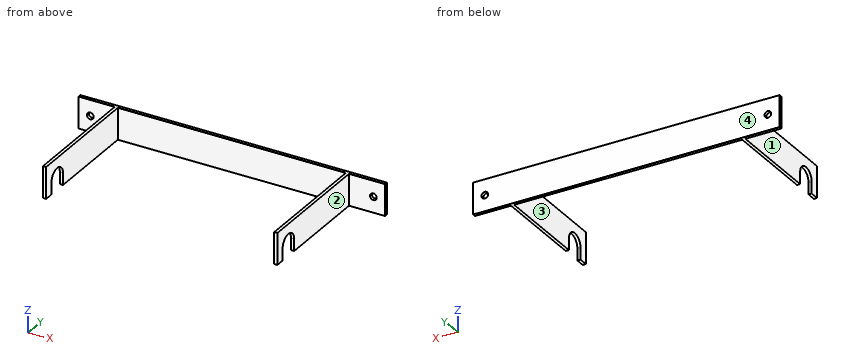
```python
from build123d import *

# Parameters (mm, degrees)
F0_W     = 390
F0_H     = 40
F0_R     = 4.25
F1_DEPTH = 4
F2_W     = 4
F2_H     = 40
F3_DEPTH = 155
F5_DEPTH = 298


with BuildPart() as f1:
    # F0 (on Front) → F1 (new body)
    with BuildSketch(Plane.XZ):
        with Locations((195, 20)):
            Rectangle(F0_W, F0_H)
        with Locations((15, 20)):
            Circle(F0_R, mode=Mode.SUBTRACT)
        with Locations((375, 20)):
            Circle(F0_R, mode=Mode.SUBTRACT)
    extrude(amount=F1_DEPTH)

    # F2 (on face) → F3 (join)
    with BuildSketch(Plane.XZ.offset(4)):
        with Locations((48, 20)):
            Rectangle(F2_W, F2_H)
        with Locations((342, 20)):
            Rectangle(F2_W, F2_H)
    extrude(amount=F3_DEPTH)

    # F4 (on face) → F5 (cut, through all)
    with BuildSketch(Plane.YZ.offset(344)):
        with BuildLine():
            Line((-122.5, 0), (-122.5, 15))
            ThreePointArc((-122.5, 15), (-135, 27.5), (-147.5, 15))
            Line((-147.5, 15), (-147.5, 0))
            Line((-147.5, 0), (-122.5, 0))
        make_face()
    extrude(amount=-F5_DEPTH, mode=Mode.SUBTRACT)


solid = f1.part
```
Part model, mm, in its own coordinate system. Face numbers are marked on the shaded views. A direction names the side the tool comes from. Round coordinates to 2 decimals unless told otherwise and drop trailing zeros. Order: outer loops, then holes, each group sorted by start corner. A loop starts at its lowest first (then second) coordinate and runs counter-clockwise, first axis right, second up. Notation, with made-up numbers: M 35,40.25 L 52,40.25 A28 ccw 52,59.25 Z; hole C 34,41.5 d10. An arc over 180 degrees is marked long. Answer in a Markdown table with one row per item. Add a question column.
Q1. Cut at D-D on z = 32. Give the cut face in (x, y), and give its area (3 significant figures).
Q2. Cut at A-A on y = -135. Give the cut face in (x, z), and give its area (3 significant figures).
Q3. Pin check, flat tips, straight feed: pin 1 (7.5 mm diameter, centred on x = 15, z = 20, fed in from +Y); pin 2 (10 mm diameter, centred on x = 198, z = 16.5, fed in from -Y); pin 3 (6 mm diameter, centred on y = -123, z = 10.5, fed in from -X); pin 4 (20 mm diameter, centred on y = -82, z = 19.5, fed in from +X). Stop position of each tip, or through.
Q4. 3-axis set-ups, long thin cutter, end or side, ignore diameter. For the marked faces 1, 2, 3 and 4: which of +Z, -Z, +X, -X, +Y, -Y reach the whole face in a straight line?
Q5. Cut at B-B on x = 15. Give the cut face in (y, z), and give its area (3 significant figures).
Q6. Cut at C-C on z = 11.5. Give the cut face in (x, y).
Q7. Wall check: L1, parallel to X at y = -22.5, z = 32; L2, parallel to Z at x = 15, y = -1.85; L3, parallel to Y at x = 56, z = 26. Give the ranges that are in metal, low to high. Write a range as from..to.
Established:
| question | item | result |
|---|---|---|
| 1 | outline | M 0,-4 L 46,-4 L 46,-159 L 50,-159 L 50,-4 L 340,-4 L 340,-159 L 344,-159 L 344,-4 L 390,-4 L 390,0 L 0,0 Z |
| 1 | area | 2,800 mm2 |
| 2 | outline | M 46,27.5 L 50,27.5 L 50,40 L 46,40 Z; M 340,27.5 L 344,27.5 L 344,40 L 340,40 Z |
| 2 | area | 100 mm2 |
| 3 | pin 1 | passes through |
| 3 | pin 2 | stops at y = -4 |
| 3 | pin 3 | stops at x = 46 |
| 3 | pin 4 | stops at x = 344 |
| 4 | face 1 | +Z, -Z, -X, -Y |
| 4 | face 2 | +Z, -Z, +X, -Y |
| 4 | face 3 | +Z, -Z, -Y |
| 4 | face 4 | +Z, -Z, +X, -X, +Y |
| 5 | outline | M -4,0 L 0,0 L 0,15.75 L -4,15.75 Z; M -4,24.25 L 0,24.25 L 0,40 L -4,40 Z |
| 5 | area | 126 mm2 |
| 6 | outline | M 0,-4 L 46,-4 L 46,-122.5 L 50,-122.5 L 50,-4 L 340,-4 L 340,-122.5 L 344,-122.5 L 344,-4 L 390,-4 L 390,0 L 0,0 Z; M 46,-159 L 50,-159 L 50,-147.5 L 46,-147.5 Z; M 340,-159 L 344,-159 L 344,-147.5 L 340,-147.5 Z |
| 7 | L1 | x = 46..50, 340..344 |
| 7 | L2 | z = 0..15.75, 24.25..40 |
| 7 | L3 | y = -4..0 |
